```python
from build123d import *

# Parameters (mm, degrees)
SKETCH1_R           = 55
BOSS_EXTRUDE1_DEPTH = 40
SHELL1_T            = -5
SKETCH2_R           = 35
CUT_EXTRUDE1_DEPTH  = 86.293610546
SKETCH3_R           = 2
CUT_EXTRUDE2_DEPTH  = 88.464278423
BOSS_EXTRUDE2_START = 10
SKETCH4_R           = 55
SKETCH4_R_2         = 35
SKETCH4_R_3         = 4.1
SKETCH4_R_4         = 2
BOSS_EXTRUDE2_DEPTH = 10
SKETCH5_R           = 4.1
CUT_EXTRUDE3_DEPTH  = 93.466210045
CUT_EXTRUDE4_DEPTH  = 9


with BuildPart() as part:
    # Sketch1 → Boss-Extrude1 (new body)
    with BuildSketch(Plane(origin=(0, 0, 0), x_dir=(1, 0, 0), z_dir=(0, 1, 0))):
        with Locations(Location((0, 0, 0), (0, 0, 270))):
            Circle(SKETCH1_R)
    extrude(amount=BOSS_EXTRUDE1_DEPTH)

    # Shell1
    shell1_openings = [part.faces().sort_by_distance(p)[0] for p in [
        (0, 0, 0),
    ]]
    offset(amount=SHELL1_T, openings=shell1_openings, kind=Kind.INTERSECTION)

    # Sketch2 → Cut-Extrude1 (cut, through all)
    with BuildSketch(Plane.XZ.offset(-35)):
        with Locations(Location((0, 0, 0), (0, 0, 270))):
            Circle(SKETCH2_R)
    extrude(amount=-CUT_EXTRUDE1_DEPTH, mode=Mode.SUBTRACT)

    # Sketch3 → Cut-Extrude2 (cut, through all)
    with BuildSketch(Plane(origin=(0, 40, 0), x_dir=(1, 0, 0), z_dir=(0, 1, 0))):
        with Locations(Location((-20, -34.641016151, 0), (0, 0, 270))):
            Circle(SKETCH3_R)
        with Locations(Location((-20, 34.641016151, 0), (0, 0, 270))):
            Circle(SKETCH3_R)
        with Locations(Location((20, 34.641016151, 0), (0, 0, 270))):
            Circle(SKETCH3_R)
        with Locations(Location((20, -34.641016151, 0), (0, 0, 270))):
            Circle(SKETCH3_R)
    extrude(amount=-CUT_EXTRUDE2_DEPTH, mode=Mode.SUBTRACT)

    # Sketch4 → Boss-Extrude2 (add)
    with BuildSketch(Plane(origin=(0, 40, 0), x_dir=(1, 0, 0), z_dir=(0, 1, 0)).offset(BOSS_EXTRUDE2_START)):
        with Locations(Location((0, 0, 0), (0, 0, 270))):
            Circle(SKETCH4_R)
        with Locations(Location((0, 0, 0), (0, 0, 90))):
            Circle(SKETCH4_R_2, mode=Mode.SUBTRACT)
        with Locations(Location((-33.591727055, -32.872418126, 0), (0, 0, 270))):
            Circle(SKETCH4_R_3, mode=Mode.SUBTRACT)
        with Locations(Location((-33.591727055, 32.872418126, 0), (0, 0, 270))):
            Circle(SKETCH4_R_3, mode=Mode.SUBTRACT)
        with Locations(Location((33.591727055, 32.872418126, 0), (0, 0, 270))):
            Circle(SKETCH4_R_3, mode=Mode.SUBTRACT)
        with Locations(Location((33.591727055, -32.872418126, 0), (0, 0, 270))):
            Circle(SKETCH4_R_3, mode=Mode.SUBTRACT)
        with Locations(Location((20, 34.641016151, 0), (0, 0, 270))):
            Circle(SKETCH4_R_4, mode=Mode.SUBTRACT)
        with Locations(Location((20, -34.641016151, 0), (0, 0, 270))):
            Circle(SKETCH4_R_4, mode=Mode.SUBTRACT)
        with Locations(Location((-20, -34.641016151, 0), (0, 0, 270))):
            Circle(SKETCH4_R_4, mode=Mode.SUBTRACT)
        with Locations(Location((-20, 34.641016151, 0), (0, 0, 270))):
            Circle(SKETCH4_R_4, mode=Mode.SUBTRACT)
    extrude(amount=-BOSS_EXTRUDE2_DEPTH)

    # Sketch5 → Cut-Extrude3 (cut, through all)
    with BuildSketch(Plane(origin=(0, 50, 0), x_dir=(1, 0, 0), z_dir=(0, 1, 0))):
        with Locations(Location((-33.591727055, -32.872418126, 0), (0, 0, 179.732355429))):
            Circle(SKETCH5_R)
        with Locations(Location((-33.591727055, 32.872418126, 0), (0, 0, 90.972475399))):
            Circle(SKETCH5_R)
        with Locations(Location((33.591727055, 32.872418126, 0), (0, 0, 89.027524601))):
            Circle(SKETCH5_R)
        with Locations(Location((33.591727055, -32.872418126, 0), (0, 0, 0.267644571))):
            Circle(SKETCH5_R)
    extrude(amount=-CUT_EXTRUDE3_DEPTH, mode=Mode.SUBTRACT)

    # Sketch6 → Cut-Extrude4 (cut)
    with BuildSketch(Plane(origin=(0, 50, 0), x_dir=(1, 0, 0), z_dir=(0, 1, 0))):
        Polygon((37.266727055, -26.507131408), (29.916727055, -26.507131408), (26.241727055, -32.872418126), (29.916727055, -39.237704844), (37.266727055, -39.237704844), (40.941727055, -32.872418126), align=None)
        Polygon((-28.521851271, -38.19396485), (-26.448194513, -31.142550265), (-31.518070297, -25.821003541), (-38.661602839, -27.550871402), (-40.735259598, -34.602285987), (-35.665383814, -39.923832711), align=None)
        Polygon((-26.241727055, 32.872418126), (-29.916727055, 39.237704844), (-37.266727055, 39.237704844), (-40.941727055, 32.872418126), (-37.266727055, 26.507131408), (-29.916727055, 26.507131408), align=None)
        Polygon((31.518070297, 25.821003541), (38.661602839, 27.550871402), (40.735259598, 34.602285987), (35.665383814, 39.923832711), (28.521851271, 38.19396485), (26.448194513, 31.142550265), align=None)
    extrude(amount=-CUT_EXTRUDE4_DEPTH, mode=Mode.SUBTRACT)


solid = part.part
```
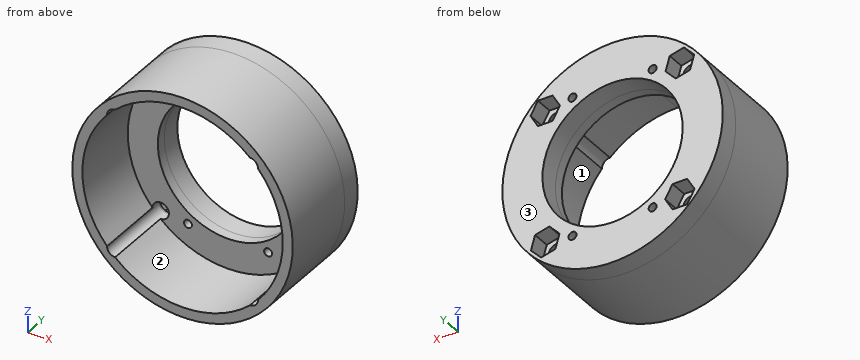
Build history of the part. All positions in model axes, mm. Face numbers are marked on the shaded views. Give positions to 0.01 mm unless a question says otherwise; leave off trailing zeros. Order: outer loops, then holes, each group sorted by start corner. A loop starts at its lowest first (then second) coordinate and runs counter-clockwise, first axis right, second up. Notation, with made-up numbers: M 82,80 L 102,80 A27 cw 102,105 Z; hole C 82.25,58.25 d1. An arc over 180 degrees is marked long. Return JSON: item names as keys, results as strings.
Q1. Band-saw the part on A-A (z = 0). Give the cut face in (x, y).
Answer list:
{"outline": "M -55,0 L -50,0 L -50,35 L -35,35 L -35,50 L -55,50 Z; M 35,35 L 50,35 L 50,0 L 55,0 L 55,50 L 35,50 Z"}
Q2. Wall check: probe 1 along X at (y, z) = (29, -1.5); probe 2 along X at (y, z) = (38, 0); probe 3 along Y at (x, z) = (19.5, -38.5). Give the ranges that are in metal, low to high. Write a range as from..to.
Answer list:
{"probe 1": "x = -54.98..-49.98, 49.98..54.98", "probe 2": "x = -55..-35, 35..55", "probe 3": "y = 35..50"}
Q3. Band-saw the part on B-B (y = 28.5). Give the cut face in (x, z).
Answer list:
{"outline": "C 0,0 d110; hole M -37.69,-32.85 A4.1 ccw -33.66,-36.97 A50 ccw 33.66,-36.97 A4.1 ccw 37.69,-32.85 A50 ccw 37.69,32.85 A4.1 ccw 33.66,36.97 A50 ccw -33.66,36.97 A4.1 ccw -37.69,32.85 A50 ccw Z"}
Q4. Band-saw the part on D-D (y = 38.5). Count the separate pieces of the cut face and the enclosed holes in it, then the cut area to 3 significant figures.
Answer list:
{"separate pieces": "1", "enclosed holes": "9", "area": "5,390 mm^2"}
Q5. Two-plate mould, pull along Z, no slides. Class the marked faces 1, 2 and 3: pulls with the +Z half, pulls with the -Z half, needs draft (parallel to the pull), parting line crosses it, or undercut.
Answer list:
{"face 1": "undercut", "face 2": "undercut", "face 3": "needs draft"}
Q6. Band-saw the part on C-C (x = 9). Give the cut face in (y, z), then the cut area to 3 significant figures.
Answer list:
{"outline": "M 0,-54.26 L 50,-54.26 L 50,-33.82 L 35,-33.82 L 35,-49.18 L 0,-49.18 Z; M 0,49.18 L 35,49.18 L 35,33.82 L 50,33.82 L 50,54.26 L 0,54.26 Z", "area": "968 mm^2"}
Q7. Flat gauge pins, fed straight in: pin 1 (7.5 mm diameter, centred on x = 33.59, z = 32.87, fed in from +Y); pin 2 (9.5 mm diameter, centred on x = 33.59, z = 32.87, fed in from +Y); pin 3 (3 mm diameter, centred on y = 26.5, z = -23.5, fed in from -X); pin 4 (1 mm diameter, centred on y = 40, z = 5.5, fed in from +X). Where does each tip first touch, or does it go through?
Answer list:
{"pin 1": "passes through", "pin 2": "stops at y = 41", "pin 3": "stops at x = -50.41", "pin 4": "stops at x = 54.77"}
